Model file for the job. Use its own axes, mm. A direction names the side the tool comes from. Coordinates: 2 decimals unless noted, no trailing zeros. Write each loop counter-clockwise with the first axis right and the second up, starting at its lowest first coordinate (ties: lowest second). Pieces come first, ordered by that corner, then holes. Notation, with made-up numbers: (20.5, 8) -> (51.5, 8) arc R26 ccw to (51.5, 24) -> close; hole circle Ø4 at (73.25, 20.25). An arc over 180 degrees is marked (long way). Answer as a JSON object with one key per item and string values. Group by question number.
from build123d import *

# Parameters (mm, degrees)
F0_W     = 307.975
F0_H     = 609.6
F1_DEPTH = 914.4
F2_T     = -12.7
F3_W     = 28.575
F3_H     = 19.05
F3_W_2   = 4.7625
F4_DEPTH = 19.05
F3_W_3   = 225.425
F3_H_2   = 395.2875
F3_W_4   = 177.8
F3_H_3   = 334.9625
F5_DEPTH = 19.05
F6_W     = 7.9375
F6_H     = 334.9625
F7_DEPTH = 177.8


with BuildPart() as f1:
    # F0 (on Top) → F1 (new body)
    with BuildSketch(Plane.XY):
        Rectangle(F0_W, F0_H)
    extrude(amount=F1_DEPTH)

    # F2
    f2_openings = [f1.faces().sort_by_distance(p)[0] for p in [
        (0, -304.8, 457.2),
    ]]
    offset(amount=F2_T, openings=f2_openings)

    # F3 (on face) → F4 (join)
    with BuildSketch(Plane.XZ.offset(304.8)):
        Polygon((-141.2875, 901.7), (-141.2875, 477.8375), (-112.7125, 477.8375), (-112.7125, 873.125), (112.7125, 873.125), (112.7125, 477.8375), (141.2875, 477.8375), (141.2875, 901.7), align=None)
        Polygon((-153.9875, 914.4), (-153.9875, 477.8375), (-146.05, 477.8375), (-146.05, 908.05), (146.05, 908.05), (146.05, 477.8375), (153.9875, 477.8375), (153.9875, 914.4), align=None)
        Polygon((-112.7125, 436.5625), (-141.2875, 436.5625), (-141.2875, 12.7), (141.2875, 12.7), (141.2875, 436.5625), (112.7125, 436.5625), (112.7125, 41.275), (-112.7125, 41.275), align=None)
        Polygon((-146.05, 436.5625), (-153.9875, 436.5625), (-153.9875, 0), (153.9875, 0), (153.9875, 436.5625), (146.05, 436.5625), (146.05, 6.35), (-146.05, 6.35), align=None)
        Polygon((-141.2875, 436.5625), (-146.05, 436.5625), (-146.05, 6.35), (146.05, 6.35), (146.05, 436.5625), (141.2875, 436.5625), (141.2875, 12.7), (-141.2875, 12.7), align=None)
        with Locations((-127, 446.0875)):
            Rectangle(F3_W, F3_H)
        Polygon((-153.9875, 477.8375), (-153.9875, 436.5625), (-146.05, 436.5625), (-146.05, 455.6125), (-141.2875, 455.6125), (-141.2875, 458.7875), (-146.05, 458.7875), (-146.05, 477.8375), align=None)
        with Locations((-143.66875, 446.0875)):
            Rectangle(F3_W_2, F3_H)
        with Locations((-127, 468.3125)):
            Rectangle(F3_W, F3_H)
        with Locations((127, 468.3125)):
            Rectangle(F3_W, F3_H)
        with Locations((127, 446.0875)):
            Rectangle(F3_W, F3_H)
        Polygon((146.05, 436.5625), (153.9875, 436.5625), (153.9875, 477.8375), (146.05, 477.8375), (146.05, 458.7875), (141.2875, 458.7875), (141.2875, 455.6125), (146.05, 455.6125), align=None)
        with Locations((143.66875, 446.0875)):
            Rectangle(F3_W_2, F3_H)
    extrude(amount=-F4_DEPTH)

    # F3 (on face) → F5 (join)
    with BuildSketch(Plane.XZ.offset(304.8)):
        Polygon((-112.7125, 436.5625), (-141.2875, 436.5625), (-141.2875, 12.7), (141.2875, 12.7), (141.2875, 436.5625), (112.7125, 436.5625), (112.7125, 41.275), (-112.7125, 41.275), align=None)
        Polygon((-141.2875, 436.5625), (-146.05, 436.5625), (-146.05, 6.35), (146.05, 6.35), (146.05, 436.5625), (141.2875, 436.5625), (141.2875, 12.7), (-141.2875, 12.7), align=None)
        with Locations((0, 238.91875)):
            Rectangle(F3_W_3, F3_H_2)
        with Locations((0, 230.98125)):
            Rectangle(F3_W_4, F3_H_3, mode=Mode.SUBTRACT)
        with Locations((0, 446.0875)):
            Rectangle(F3_W_3, F3_H)
        with Locations((-127, 446.0875)):
            Rectangle(F3_W, F3_H)
        with Locations((127, 446.0875)):
            Rectangle(F3_W, F3_H)
        with Locations((143.66875, 446.0875)):
            Rectangle(F3_W_2, F3_H)
        with Locations((-143.66875, 446.0875)):
            Rectangle(F3_W_2, F3_H)
        Polygon((-141.2875, 901.7), (-141.2875, 477.8375), (-112.7125, 477.8375), (-112.7125, 873.125), (112.7125, 873.125), (112.7125, 477.8375), (141.2875, 477.8375), (141.2875, 901.7), align=None)
        with Locations((0, 675.48125)):
            Rectangle(F3_W_3, F3_H_2)
        with Locations((0, 683.41875)):
            Rectangle(F3_W_4, F3_H_3, mode=Mode.SUBTRACT)
        with Locations((-127, 468.3125)):
            Rectangle(F3_W, F3_H)
        with Locations((0, 468.3125)):
            Rectangle(F3_W_3, F3_H)
        with Locations((127, 468.3125)):
            Rectangle(F3_W, F3_H)
        with Locations((143.66875, 468.3125)):
            Rectangle(F3_W_2, F3_H)
        Polygon((-146.05, 908.05), (-146.05, 477.8375), (-141.2875, 477.8375), (-141.2875, 901.7), (141.2875, 901.7), (141.2875, 477.8375), (146.05, 477.8375), (146.05, 908.05), align=None)
        with Locations((-143.66875, 468.3125)):
            Rectangle(F3_W_2, F3_H)
    extrude(amount=F5_DEPTH)

    # F6 (on face) → F7 (join, through all)
    with BuildSketch(Plane(origin=(88.9, 0, 0), x_dir=(0, -1, 0), z_dir=(-1, 0, 0))):
        with Locations((313.53125, 230.98125)):
            Rectangle(F6_W, F6_H)
        with Locations((313.53125, 683.41875)):
            Rectangle(F6_W, F6_H)
    extrude(amount=F7_DEPTH)


solid = f1.part
(1) Cut at A-A on z = 436. List the corners of the cut face in (x, y), plus the area to 3 significant figures.
(2) 3-axis set-ups, long thin cutter, end or side, ignore diameter. For faces 4 (the face through (-146.05, -314, 234)), 5 (the face through (146.05, -314, 228)), 6 (the face through (141.288, -11, 451)): which of +Z, -Z, +X, -X, +Y, -Y reach the whole face in a straight line?
(3) Wall check: probe 1 along Z at (x, y) = (-130.5, 224.5); probe 2 along X at (y, z) = (-128.5, 474.5); probe 3 along Y at (x, z) = (21.5, 125). Give the ranges that are in metal, low to high.
(4) Cut at C-C on x = 125.5. List the corners of the cut face in (y, z).
(5) Cut at D-D on z = 313.5. List the corners of the cut face in (x, y), plus the area to 4 significant figures.
(6) Pin check, flat tips, straight feed: pin 1 (5 mm diameter, centred on x = -15, y = -308, fed in from -Z); pin 2 (15 mm diameter, centred on y = -310, z = 318, fed in from -X); pin 3 (7 mm diameter, centred on y = -320.5, z = 694, fed in from +X); pin 4 (5 mm diameter, centred on x = -17, y = -320.5, fed in from +Z). Stop position of each tip, or through.
(7) Pull direction Z, two halves, no side cores. Call faces 1 (the face through (-112.712, -295, 246)), 2 (the face through (-2, -314, 6.35)), 3 (the face through (-99, -323.85, 687)): released by +Z, released by -Z, zero draft, split by the parting line, or undercut.
(8) Cut at B-B on y = 250. List the corners of the cut face in (x, z).
Results found:
{
 "1": {"outline": "(-153.99, -304.8) -> (-146.05, -304.8) -> (-146.05, -323.85) -> (146.05, -323.85) -> (146.05, -304.8) -> (153.99, -304.8) -> (153.99, 304.8) -> (-153.99, 304.8) -> close; hole (-141.29, -285.75) -> (-112.71, -285.75) -> (-112.71, -304.8) -> (112.71, -304.8) -> (112.71, -285.75) -> (141.29, -285.75) -> (141.29, 292.1) -> (-141.29, 292.1) -> close", "area": "25,700 mm²"},
 "2": {"face 4": "+Z, -Z, -X, -Y", "face 5": "+Z, -Z, +X, -Y", "face 6": "none"},
 "3": {"probe 1": "z = 0 to 12.7, 901.7 to 914.4", "probe 2": "x = -153.99 to -141.29, 141.29 to 153.99", "probe 3": "y = -317.5 to -309.56, 292.1 to 304.8"},
 "4": {"outline": "(-323.85, 6.35) -> (-304.8, 6.35) -> (-304.8, 0) -> (304.8, 0) -> (304.8, 914.4) -> (-304.8, 914.4) -> (-304.8, 908.05) -> (-323.85, 908.05) -> (-323.85, 458.79) -> (-285.75, 458.79) -> (-285.75, 901.7) -> (292.1, 901.7) -> (292.1, 12.7) -> (-285.75, 12.7) -> (-285.75, 455.61) -> (-323.85, 455.61) -> close"},
 "5": {"outline": "(-153.99, -304.8) -> (-146.05, -304.8) -> (-146.05, -323.85) -> (-88.9, -323.85) -> (-88.9, -317.5) -> (88.9, -317.5) -> (88.9, -323.85) -> (146.05, -323.85) -> (146.05, -304.8) -> (153.99, -304.8) -> (153.99, 304.8) -> (-153.99, 304.8) -> close; hole (-141.29, -285.75) -> (-112.71, -285.75) -> (-112.71, -304.8) -> (-88.9, -304.8) -> (-88.9, -309.56) -> (88.9, -309.56) -> (88.9, -304.8) -> (112.71, -304.8) -> (112.71, -285.75) -> (141.29, -285.75) -> (141.29, 292.1) -> (-141.29, 292.1) -> close", "area": "23,750 mm²"},
 "6": {"pin 1": "stops at z = 6.35", "pin 2": "stops at x = -153.99", "pin 3": "stops at x = 146.05", "pin 4": "stops at z = 908.05"},
 "7": {"face 1": "undercut", "face 2": "released by -Z", "face 3": "zero draft"},
 "8": {"outline": "(-153.99, 0) -> (153.99, 0) -> (153.99, 914.4) -> (-153.99, 914.4) -> close; hole (-141.29, 12.7) -> (141.29, 12.7) -> (141.29, 901.7) -> (-141.29, 901.7) -> close"}
}
